Autodesk Inventor part; units mm, degrees
ref_plane "YZ Plane" through (0, 0, 0) normal (1, 0, 0) x (0, 1, 0)
ref_plane "XZ Plane" through (0, 0, 0) normal (0, 1, 0) x (-1, 0, 0)
ref_plane "XY Plane" through (0, 0, 0) normal (0, 0, 1) x (1, 0, 0)
sketch "Sketch1" plane through (0, 0, 0) normal (0, 0, 1) x (1, 0, 0)
  circle A0 centre (0, 0) radius 2.5
  line L0 (-13, 13) -> (13, 13)
  line L1 (13, 13) -> (13, -13)
  line L2 (13, -13) -> (-13, -13)
  line L3 (-13, -13) -> (-13, 13)
  line L4 (-13, 13) -> (13, -13) construction
  line L5 (13, 13) -> (-13, -13) construction
  dimension "d0" = 5
  dimension "d1" = 26
  dimension "d2" = 26
extrude "Extrusion1" add sketch "Sketch1" against normal blind 10 contours A0
extrude "Extrusion2" add sketch "Sketch1" along normal blind 4 contours A0 | L0 L1 L2 L3
properties part number "corredor"
The model under review builds one solid part; all positions refer to its coordinate system, in mm. A direction names the side the tool comes from. Round coordinates to 2 decimals unless told otherwise and drop trailing zeros. Loops run counter-clockwise (first coordinate to the right, second up) from the corner with the lowest first, then second, coordinate; pieces in that order, holes last.
Item 1: Take a section at A-A (y = -1.5). Write out the cut boundary in (x, z).
Determined:
outline: (-13, 0) - (-2, 0) - (-2, -10) - (2, -10) - (2, 0) - (13, 0) - (13, 4) - (-13, 4) - close
Item 2: Take a section at C-C (z = -5.75). Write out the cut boundary in (x, y), then the cut area to 3 significant figures.
Determined:
outline: circle Ø5 at (0, 0)
area: 19.6 mm2
Item 3: Take a section at D-D (x = -10). Write out the cut boundary in (y, z), then the cut area to 3 significant figures.
Determined:
outline: (-13, 0) - (13, 0) - (13, 4) - (-13, 4) - close
area: 104 mm2
Item 4: Clearance check with flat-ended pins moving along their axes: pin 1 Ø1.5 at (y, z) = (0.5, -6.5) entering from -X; pin 2 Ø6 at (x, z) = (-4.5, -3.5) entering from +Y; pin 3 Ø4 at (x, y) = (-8, -2) entering from -Z. State where each tip first meets the part, or that it passes through.
Determined:
pin 1: stops at x = -2.5
pin 2: stops at y = 2
pin 3: stops at z = 0
Item 5: Take a section at B-B (x = 0). Write out the cut boundary in (y, z).
Determined:
outline: (-13, 0) - (-2.5, 0) - (-2.5, -10) - (2.5, -10) - (2.5, 0) - (13, 0) - (13, 4) - (-13, 4) - close
Item 6: For line 1 (Z direction, x = -8.75, y = -1.5); line 2 (Y direction, x = 2.25, z = -1.5); line 3 (X direction, y = -0.25, z = -2.75), list the stretches that pass through material, from the lowest coordinate up.
Determined:
line 1: z = 0 to 4
line 2: y = -1.09 to 1.09
line 3: x = -2.49 to 2.49
Item 7: For faces 1 (the face through (0, 13, 2)), 2 (the face through (-0.54, -2.44, -4.93)), list the 3-axis set-ups (+Z, -Z, +X, -X, +Y, -Y) from which the entire face can be reached by the end or side of a thin tool; tool diameter is ignored.
Determined:
face 1: +Z, -Z, +X, -X, +Y
face 2: -Z
